Read the model definition and answer for the solid it produces. Units are mm, in the model's axes. Face numbers are marked on the shaded views. Give positions to 0.01 mm unless a question says otherwise; leave off trailing zeros. Order: outer loops, then holes, each group sorted by start corner. A loop starts at its lowest first (then second) coordinate and runs counter-clockwise, first axis right, second up. Notation, with made-up numbers: (67, 60) - (74, 60) arc R25 ccw to (74, 85) - close; hole circle Ø3 at (75, -39.75). An arc over 180 degrees is marked (long way). Write item = value, one per line.
```python
from build123d import *

# Parameters (mm, degrees)
BOSS_EXTRUDE1_DEPTH = 100
BOSS_EXTRUDE2_DEPTH = 5
CHAMFER1_SIZE       = 5
SKETCH4_W           = 30
SKETCH4_H           = 3.762328583
BOSS_EXTRUDE3_DEPTH = 30


with BuildPart() as part:
    # Sketch2 → Boss-Extrude1 (new body)
    with BuildSketch(Plane(origin=(0, 0, 0), x_dir=(0, 0, -1), z_dir=(1, 0, 0))):
        with BuildLine():
            Line((175, 0), (180, 0))
            ThreePointArc((180, 0), (127.279220614, -127.279220614), (0, -180))
            Line((0, -180), (0, -175))
            ThreePointArc((0, -175), (123.743686708, -123.743686708), (175, 0))
        make_face()
    extrude(amount=BOSS_EXTRUDE1_DEPTH)

    # Sketch3 → Boss-Extrude2 (add)
    with BuildSketch(Plane(origin=(100, 0, 0), x_dir=(0, 0, -1), z_dir=(1, 0, 0))):
        with BuildLine():
            Line((0, 0), (0, -180))
            ThreePointArc((0, -180), (127.279220614, -127.279220614), (180, 0))
            Line((180, 0), (0, 0))
        make_face()
    extrude(amount=BOSS_EXTRUDE2_DEPTH)

    # Chamfer1
    # the kernel refuses this chamfer: 20, 5 mm, written as the material it takes off along each edge
    with BuildSketch(Plane(origin=(-80.427863616, -175, 0), x_dir=(0, -1, 0), z_dir=(1, 0, 0))) as chamfer1_piece_1:
        with BuildLine():
            Line((CHAMFER1_SIZE, 0), (-2.813534961, 31.254139845))
            ThreePointArc((-2.813534961, 31.254139845), (-0.740839573, 16.085552754), (0, 0))
            Line((0, 0), (CHAMFER1_SIZE, 0))
        make_face()
    extrude(amount=180.427863616, mode=Mode.SUBTRACT)

    # Sketch4 → Boss-Extrude3 (add)
    with BuildSketch(Plane.ZY.offset(-100)):
        with Locations((-160, -1.881164292)):
            Rectangle(SKETCH4_W, SKETCH4_H)
    extrude(amount=BOSS_EXTRUDE3_DEPTH)


solid = part.part
```
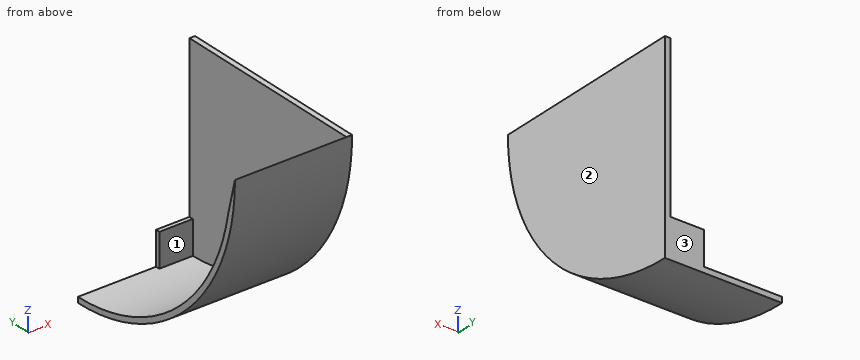
1. Section C-C (z = -154) is taken. Determine the outline of the cut face in (x, y).
Recorded:
outline = (0, -93.19) - (105, -93.19) - (105, 0) - (70, 0) - (70, -3.76) - (100, -3.76) - (100, -83.12) - (0, -83.12) - close
2. Determine the mould class of the marked faces 1, 2 and 3 for opening direction Y: +Y half, -Y half, draft (parallel to the pull), parting line (faces both ways), or undercut.
Recorded:
face_1 = undercut
face_2 = draft
face_3 = +Y half
3. Section B-B (y = -97) is taken. Determine the outline of the cut face in (x, z).
Recorded:
outline = (0, -151.63) - (105, -151.63) - (105, 0) - (100, 0) - (100, -145.66) - (0, -145.66) - close
4. Straight lines are drawn through the part: L1, parallel to X at y = -143, z = -10; L2, parallel to Y at x = 89, z = -160.5; L3, parallel to Z at x = 51.5, y = -114.5. For each, find the intervals that lie inside material, in ascending order. Write a range as [from, to].
Recorded:
L1 = [100, 105]
L2 = [-81.48, -69.75], [-3.76, 0]
L3 = [-138.89, -132.34]
5. Section A-A (x = 93) is taken. Determine the outline of the cut face in (y, z), and give its area (3 significant figures).
Recorded:
outline = (-180, 0) arc R180 ccw to (0, -180) - (0, -145) - (-3.76, -145) - (-3.76, -174.96) arc R175 cw to (-172.19, -31.25) - close
area = 1,440 mm^2
6. Flat-ended cylindrical pins translate along their axes: pin 1 (1.5 mm diameter, centred on x = 18, y = -61.5, fed in from -Z); pin 2 (6 mm diameter, centred on y = -71.5, z = -107, fed in from -X); pin 3 (6 mm diameter, centred on x = 27, y = -123, fed in from +Z). Find the tip coordinate at first contact, or state that the pin passes through.
Recorded:
pin_1 = -169.44
pin_2 = 100
pin_3 = -121.45
7. Section D-D (x = 29) is taken. Determine the outline of the cut face in (y, z), and give its area (3 significant figures).
Recorded:
outline = (-180, 0) arc R180 ccw to (0, -180) - (0, -175) arc R175 cw to (-172.19, -31.25) - close
area = 1,330 mm^2
